from build123d import *

# Parameters (mm, degrees)
F0_R     = 1.5875
F1_DEPTH = 3.175
F2_R     = 26.9875
F2_R_2   = 26.19375
F3_DEPTH = 3.175
F4_R     = 3.175
F5_DEPTH = 3.175


with BuildPart() as f1:
    # F0 (on Top) → F1 (new body)
    with BuildSketch(Plane.XY):
        with BuildLine():
            Line((36.5125, 3.175), (29.994929, 3.175))
            ThreePointArc((29.994929, 3.175), (21.328108, 21.328108), (3.175, 29.994929))
            Line((3.175, 29.994929), (3.175, 36.5125))
            ThreePointArc((3.175, 36.5125), (0, 39.6875), (-3.175, 36.5125))
            Line((-3.175, 36.5125), (-3.175, 29.994929))
            ThreePointArc((-3.175, 29.994929), (-21.328108, 21.328108), (-29.994929, 3.175))
            Line((-29.994929, 3.175), (-30.1625, 3.175))
            Line((-30.1625, 3.175), (-36.5125, 3.175))
            ThreePointArc((-36.5125, 3.175), (-39.6875, 0), (-36.5125, -3.175))
            Line((-36.5125, -3.175), (-30.1625, -3.175))
            Line((-30.1625, -3.175), (-29.994929, -3.175))
            ThreePointArc((-29.994929, -3.175), (-21.328108, -21.328108), (-3.175, -29.994929))
            Line((-3.175, -29.994929), (-3.175, -36.5125))
            ThreePointArc((-3.175, -36.5125), (0, -39.6875), (3.175, -36.5125))
            Line((3.175, -36.5125), (3.175, -29.994929))
            ThreePointArc((3.175, -29.994929), (21.328108, -21.328108), (29.994929, -3.175))
            Line((29.994929, -3.175), (36.5125, -3.175))
            ThreePointArc((36.5125, -3.175), (39.6875, 0), (36.5125, 3.175))
        make_face()
        with Locations((0, -36.5125)):
            Circle(F0_R, mode=Mode.SUBTRACT)
        with Locations((-36.5125, 0)):
            Circle(F0_R, mode=Mode.SUBTRACT)
        with Locations((36.5125, 0)):
            Circle(F0_R, mode=Mode.SUBTRACT)
        with Locations((0, 36.5125)):
            Circle(F0_R, mode=Mode.SUBTRACT)
    extrude(amount=F1_DEPTH)

    # F2 (on face) → F3 (join)
    with BuildSketch(Plane.XY.offset(3.175)):
        Circle(F2_R)
        Circle(F2_R_2, mode=Mode.SUBTRACT)
    extrude(amount=F3_DEPTH)

    # F4 (on face) → F5 (cut)
    with BuildSketch(Plane.XY.offset(3.175)):
        with BuildLine():
            ThreePointArc((-2.38125, 4.124446), (0, 4.7625), (2.38125, 4.124446))
            Line((2.38125, 4.124446), (12.22375, 21.172156))
            ThreePointArc((12.22375, 21.172156), (0, 24.4475), (-12.22375, 21.172156))
            Line((-12.22375, 21.172156), (-2.38125, 4.124446))
        make_face()
        Circle(F4_R)
        with BuildLine():
            ThreePointArc((4.7625, 0), (4.124446, -2.38125), (2.38125, -4.124446))
            Line((2.38125, -4.124446), (12.22375, -21.172156))
            ThreePointArc((12.22375, -21.172156), (21.172156, -12.22375), (24.4475, 0))
            Line((24.4475, 0), (4.7625, 0))
        make_face()
        with BuildLine():
            Line((-4.7625, 0), (-24.4475, 0))
            ThreePointArc((-24.4475, 0), (-21.172156, -12.22375), (-12.22375, -21.172156))
            Line((-12.22375, -21.172156), (-2.38125, -4.124446))
            ThreePointArc((-2.38125, -4.124446), (-4.124446, -2.38125), (-4.7625, 0))
        make_face()
    extrude(amount=-F5_DEPTH, mode=Mode.SUBTRACT)


solid = f1.part
Design review of the part built by this model. Coordinates are the model's own, in mm. A direction names the side the tool comes from. Round coordinates to 2 decimals unless told otherwise and drop trailing zeros. Order: outer loops, then holes, each group sorted by start corner. A loop starts at its lowest first (then second) coordinate and runs counter-clockwise, first axis right, second up. Notation, with made-up numbers: M 9,70 L 67,70 A15 ccw 67,85 Z; hole C 53,56.25 d4. An arc over 180 degrees is marked long. Answer as CSV lines item,"result". Start each with the question number.
1) Tool access review of faces 1 (the face through (21.124, -21.53, 1.565)), 2 (the face through (-0.035, 4.762, 1.61)), 3 (the face through (-3.175, -33, 2)): name each direction out of +Z, -Z, +X, -X, +Y, -Y from which nothing blocks a thin tool from reaching the whole face with its end or side.
2) Add section B-B (x = -9). Give the boundary of the cut face in (y, z) (3 decimals).
3) Add section D-D (z = 5). Give the boundary of the cut face in (x, y) (1 decimal), then the cut area to 3 significant figures.
4) For pin 1 Ø3 at (x, z) = (-11.5, 5) entering from -Y; pin 2 Ø1.5 at (x, y) = (-5.5, -10) entering from +Z (3 decimals); pin 3 Ø2.5 at (x, z) = (32, 1) entering from +Y (3 decimals), all flat-tipped, find the tip position at first contact; note any pin that passes through.
5) Add section A-A (x = 0). Give the number of separate pieces and of enclosed holes in the cut face, then the cut area to 3 significant figures.
6) Wall thickness on line 1 along Y through (x, z) = (0, 0.95) (1 decimal); line 2 along X through (y, z) = (1, 4.5); line 3 along Y through (x, z) = (0.5, 2): over which ranges is each line inside the solid? List them lowest first. Write a range as [from, to].
7) Add section C-C (y = -9). Give the boundary of the cut face in (x, z) (3 decimals), then the cut area to 3 significant figures.
8) The part is to be moulded in two halves that separate along Y. For faces 4 (the face through (39.687, -0.07, 1.565)), 5 (the face through (-5.68, -25.57, 4.74)), 6 (the face through (-21.124, 21.53, 1.565)), 7 (the face through (3.175, 33, 2)), say which applies: +Y half, -Y half, draft (parallel to the pull), parting line (faces both ways), or undercut.
Resolved:
1,face 1,"+Z, -Z, +X, -Y"
1,face 2,"+Z, -Z"
1,face 3,"+Z, -Z, -X, -Y"
2,outline,"M -28.788,0 L -15.588,0 L -15.588,3.175 L -24.599,3.175 L -24.599,6.35 L -25.443,6.35 L -25.443,3.175 L -28.788,3.175 Z; M 0,0 L 15.588,0 L 15.588,3.175 L 0,3.175 Z; M 22.731,0 L 28.788,0 L 28.788,3.175 L 25.443,3.175 L 25.443,6.35 L 24.599,6.35 L 24.599,3.175 L 22.731,3.175 Z"
3,outline,"C 0,0 d54; hole C 0,0 d52.4"
3,area,"133 mm^2"
4,pin 1,"y = -25.07"
4,pin 2,"z = 3.175"
4,pin 3,"y = 3.175"
5,separate pieces,"5"
5,enclosed holes,"0"
5,area,"154 mm^2"
6,line 1,"[-39.7, -38.1], [-34.9, -3.2], [3.2, 4.8], [24.4, 34.9], [38.1, 39.7]"
6,line 2,"[-26.97, -26.17], [26.17, 26.97]"
6,line 3,"[-39.65, -38.02], [-35.01, -3.14], [3.14, 4.74], [24.44, 35.01], [38.02, 39.65]"
7,outline,"M -28.788,0 L -22.731,0 L -22.731,3.175 L -24.599,3.175 L -24.599,6.35 L -25.443,6.35 L -25.443,3.175 L -28.788,3.175 Z; M -5.196,0 L 5.196,0 L 5.196,3.175 L -5.196,3.175 Z; M 22.731,0 L 28.788,0 L 28.788,3.175 L 25.443,3.175 L 25.443,6.35 L 24.599,6.35 L 24.599,3.175 L 22.731,3.175 Z"
7,area,"76.8 mm^2"
8,face 4,"parting line"
8,face 5,"undercut"
8,face 6,"+Y half"
8,face 7,"draft"
